Work out the finished part from the listing and answer in its coordinate system (mm). A direction names the side the tool comes from. Coordinates: 2 decimals unless noted, no trailing zeros. Order: outer loops, then holes, each group sorted by start corner. A loop starts at its lowest first (then second) coordinate and runs counter-clockwise, first axis right, second up. Notation, with made-up numbers: M 64,17 L 81,17 A23 cw 81,50 Z; hole C -13.75,39.25 d7. An arc over 180 degrees is marked long. Use a Markdown table: item, result.
from build123d import *

# Parameters (mm, degrees)
BASE_DEPTH         = 10
SKETCH2_W          = 80
SKETCH2_H          = 4
SHELF_DEPTH        = 60
SKETCH5_R          = 1.7
SKETCH5_W          = 23
SKETCH5_H          = 13
CUT_EXTRUDE2_DEPTH = 10


with BuildPart() as part:
    # Sketch1 → Base (new body)
    with BuildSketch(Plane.XY):
        Polygon((-48.262081784, 36.356877323), (-48.262081784, -23.643122677), (31.737918216, -23.643122677), (31.737918216, 36.356877323), (31.737918216, 66.356877323), (-48.262081784, 66.356877323), align=None)
    extrude(amount=BASE_DEPTH)

    # Sketch2 → Shelf (add)
    with BuildSketch(Plane.XY.offset(10)):
        with Locations((-8.262081784, 38.356877323)):
            Rectangle(SKETCH2_W, SKETCH2_H)
    extrude(amount=SHELF_DEPTH)

    # Sketch5 → Cut-Extrude2 (cut)
    with BuildSketch(Plane(origin=(0, 40.356877323, 0), x_dir=(1, 0, 0), z_dir=(0, 1, 0))):
        with Locations(Location((-22.437854868, -41.756424537, 0), (0, 0, 270))):
            Circle(SKETCH5_R)
        with Locations(Location((7.562145132, -41.756424537, 0), (0, 0, 270))):
            Circle(SKETCH5_R)
        with Locations((-7.437854868, -41.569973221)):
            Rectangle(SKETCH5_W, SKETCH5_H)
    extrude(amount=-CUT_EXTRUDE2_DEPTH, mode=Mode.SUBTRACT)


solid = part.part
1. Section A-A on x = 0.5 is taken. Determine the outline of the cut face in (y, z), then the cut area to 3 significant figures.
Answers below:
| item | result |
|---|---|
| outline | M -23.64,0 L 66.36,0 L 66.36,10 L 40.36,10 L 40.36,35.07 L 36.36,35.07 L 36.36,10 L -23.64,10 Z; M 36.36,48.07 L 40.36,48.07 L 40.36,70 L 36.36,70 Z |
| area | 1,090 mm² |
2. For faces 1 (the face through (-8, 38, 48.07)), 2 (the face through (-9, 54, 10)), 3 (the face through (-8, 66.357, 5)), 4 (the face through (-9, 36.357, 33)), determine the directions among +Z, -Z, +X, -X, +Y, -Y from which every point of the face is accessible in a straight line to the end or side of a thin tool.
Answers below:
| item | result |
|---|---|
| face 1 | +Y, -Y |
| face 2 | +Z, +X, -X, +Y |
| face 3 | +Z, -Z, +X, -X, +Y |
| face 4 | +Z, +X, -X, -Y |
3. Flat-ended cylindrical pins translate along their axes: P1, Ø6, axis at x = -38, y = 40, coming from the -Z side; P2, Ø1, axis at x = -0.5, z = 19, coming from the +Y side; P3, Ø5, axis at x = -33.5, y = -12, coming from the +Z side; P4, Ø4, axis at x = -20.5, z = 26, coming from the -Y side. Find the tip coordinate at first contact, or state that the pin passes through.
Answers below:
| item | result |
|---|---|
| P1 | z = 0 |
| P2 | y = 40.36 |
| P3 | z = 10 |
| P4 | y = 36.36 |
4. Find the intervals of material crossed by probe 1 along X at (y, z) = (40, 40); probe 2 along Y at (x, z) = (-36, 66); probe 3 along Z at (x, y) = (-25, 14.5), in increasing order.
Answers below:
| item | result |
|---|---|
| probe 1 | -48.26 to -18.94, 4.06 to 31.74 |
| probe 2 | 36.36 to 40.36 |
| probe 3 | 0 to 10 |
5. For a pull along Z with two mould halves and no side action, classify faces 5 (the face through (-9, 7, 10)), 6 (the face through (-20.75, 38.38, 41.54)), 7 (the face through (-48.262, 25, 9)), 8 (the face through (4.062, 38, 42)) as +Z half, -Z half, draft (parallel to the pull), parting line (faces both ways), or undercut.
Answers below:
| item | result |
|---|---|
| face 5 | +Z half |
| face 6 | undercut |
| face 7 | draft |
| face 8 | undercut |
6. Section D-D on y = 17 is taken. Determine the outline of the cut face in (x, z), then the cut area to 3 significant figures.
Answers below:
| item | result |
|---|---|
| outline | M -48.26,0 L 31.74,0 L 31.74,10 L -48.26,10 Z |
| area | 800 mm² |
7. Section B-B on z = 38 is taken. Determine the outline of the cut face in (x, y).
Answers below:
| item | result |
|---|---|
| outline | M -48.26,36.36 L -18.94,36.36 L -18.94,40.36 L -48.26,40.36 Z; M 4.06,36.36 L 31.74,36.36 L 31.74,40.36 L 4.06,40.36 Z |
8. Section C-C on x = -40 is taken. Determine the outline of the cut face in (y, z).
Answers below:
| item | result |
|---|---|
| outline | M -23.64,0 L 66.36,0 L 66.36,10 L 40.36,10 L 40.36,70 L 36.36,70 L 36.36,10 L -23.64,10 Z |
